The model under review builds one solid part; all positions refer to its coordinate system, in mm. Face numbers are marked on the shaded views. Coordinates: 2 decimals unless noted, no trailing zeros. Loops run counter-clockwise (first coordinate to the right, second up) from the corner with the lowest first, then second, coordinate; pieces in that order, holes last. Notation, with made-up numbers: M -5,35 L 52,35 A6 ccw 52,39 Z; hole C 73.25,28 d5. An arc over 180 degrees is marked long. One line per item, written item: value.
```python
from build123d import *

# Parameters (mm, degrees)
SKETCH_1_W      = 76.2
SKETCH_1_H      = 19.05
SKETCH_1_R      = 2.3876
EXTRUDE_1_DEPTH = 6.35


with BuildPart() as part:
    # 스케치1 → 보스-돌출1 (new body)
    with BuildSketch(Plane(origin=(0, 6.35, 0), x_dir=(1, 0, 0), z_dir=(0, 1, 0))):
        with Locations((-28.575, 0)):
            Rectangle(SKETCH_1_W, SKETCH_1_H)
        with Locations(Location((-57.15, 0, 0), (0, 0, 90))):
            Circle(SKETCH_1_R, mode=Mode.SUBTRACT)
        with BuildLine():
            Line((4.7498, 4.214486915), (4.7498, -4.214486915))
            ThreePointArc((4.7498, -4.214486915), (-6.35, 0), (4.7498, 4.214486915))
        make_face(mode=Mode.SUBTRACT)
    extrude(amount=-EXTRUDE_1_DEPTH)


solid = part.part
```
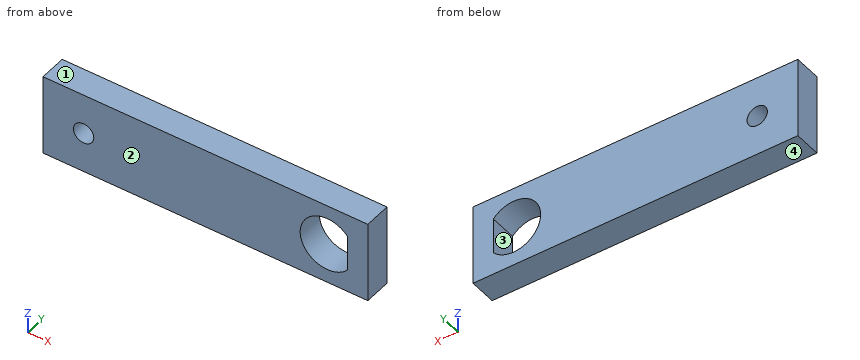
(1) Add section B-B on y = 3. State the section outline as (x, z) points (3 decimals), then the cut area to 3 significant figures.
Checks:
outline: M -66.675,-9.525 L 9.525,-9.525 L 9.525,9.525 L -66.675,9.525 Z; hole C -57.15,0 d4.775; hole M 4.75,-4.214 L 4.75,4.214 A6.35 ccw long Z
area: 1,320 mm^2
(2) Draft analysis for pull direction Z (two halves, no side actions). For the marked faces 1, 2, 3 and 4, state which applies: pulls with the +Z half, pulls with the -Z half, needs draft (parallel to the pull), parting line crosses it, or undercut.
Checks:
face 1: pulls with the +Z half
face 2: needs draft
face 3: undercut
face 4: pulls with the -Z half
(3) To check wall thickness, follow L1, parallel to X at y = 0.75, z = -0.25 (3 decimals); L2, parallel to Z at x = -57.15, y = 4.75 (3 decimals); L3, parallel to Z at x = 0, y = 4.75 (3 decimals). State the ranges of each line that lie inside material, in increasing order. Write a range as [from, to].
Checks:
L1: [-66.675, -59.524], [-54.776, -6.345], [4.75, 9.525]
L2: [-9.525, -2.388], [2.388, 9.525]
L3: [-9.525, -6.35], [6.35, 9.525]
(4) Add section C-C on z = 0. State the section outline as (x, y) points (3 decimals), then the cut area to 3 significant figures.
Checks:
outline: M -66.675,0 L -59.538,0 L -59.538,6.35 L -66.675,6.35 Z; M -54.762,0 L -6.35,0 L -6.35,6.35 L -54.762,6.35 Z; M 4.75,0 L 9.525,0 L 9.525,6.35 L 4.75,6.35 Z
area: 383 mm^2
(5) Add section A-A on x = -57.15. State the section outline as (y, z) points (3 decimals), then the cut area to 3 significant figures.
Checks:
outline: M 0,-9.525 L 6.35,-9.525 L 6.35,-2.388 L 0,-2.388 Z; M 0,2.388 L 6.35,2.388 L 6.35,9.525 L 0,9.525 Z
area: 90.6 mm^2
(6) Add section D-D on x = 0. State the section outline as (y, z) points (3 decimals), then the cut area to 3 significant figures.
Checks:
outline: M 0,-9.525 L 6.35,-9.525 L 6.35,-6.35 L 0,-6.35 Z; M 0,6.35 L 6.35,6.35 L 6.35,9.525 L 0,9.525 Z
area: 40.3 mm^2
